Input: part model. Units: mm. Frame: model coordinates. A direction names the side the tool comes from. Give positions to 0.01 mm unless a question says otherwise; leave off trailing zeros. Write each loop counter-clockwise with the first axis right and the second up, starting at its lowest first coordinate (ties: lowest second). Pieces come first, ordered by that corner, then holes. Notation, with made-up numbers: (74, -9) - (111, -9) arc R18 ccw to (111, 9) - close; hole circle Ø11 at (-0.5, 51.5). An arc over 180 degrees is marked (long way). Use a Markdown table: item, result. Add a question column.
1. Section query B-B, the plane z = -95. Return loops of the section in (x, y).
2. Mould query, pull axis X, two halves, no side actions, for faces 5 (the cylindrical face through (-22.2, 12.1, -11.5)), 6 (the cylindrical face through (0.706, 68.675, -112.466)), 7 (the flat face through (-4, 81, -84)). Classes: released by +X, released by -X, zero draft, split by the parting line, or undercut.
3. Section query A-A, the plane x = 0. Return loops of the section in (y, z), plus the area to 3 significant figures.
4. Set-up query: faces 1 (the flat face through (22, 18, 1)), 2 (the flat face through (-22, 18, 1)), 3 (the flat face through (8, 56, -103)), 4 (the flat face through (22, 9, -33.509)). Return all of +Z, -Z, +X, -X, +Y, -Y with unobstructed straight access to the full face (end or side cutting, diameter ignored); none if empty.
5. Section query D-D, the plane y = 73.5. Return loops of the section in (x, z).
6. Material intervals for probe 1 along Z at (x, y) = (14.5, 5); probe 2 along X at (y, z) = (53, -54.5); probe 3 along Y at (x, z) = (-12, -20.5), sorted ascending.
7. Section query C-C, the plane z = -5. Return loops of the section in (x, y), plus the area to 3 significant figures.
8. Pin query (flat end, axial travel): pin 1 (12 mm diameter, centred on x = 19.5, y = 68, fed in from +Z); pin 2 (15.5 mm diameter, centred on x = -22.5, z = -5.51, fed in from -Y); pin 3 (25 mm diameter, centred on x = 19, z = -3, fed in from +Y). Return the tip coordinate at first contact, or that it passes through.
```python
from build123d import *

# Parameters (mm, degrees)
SKETCH1_W           = 56
SKETCH1_H           = 18
BOSS_EXTRUDE1_DEPTH = 75
SKETCH2_R           = 6
CUT_EXTRUDE1_DEPTH  = 75
SKETCH3_W           = 32
SKETCH3_H           = 6
CUT_EXTRUDE2_DEPTH  = 75
BOSS_EXTRUDE5_DEPTH = 6
SKETCH23_R          = 18
SKETCH23_R_2        = 11
BOSS_EXTRUDE7_DEPTH = 25


with BuildPart() as part:
    # Sketch1 → Boss-Extrude1 (new body)
    with BuildSketch(Plane(origin=(0, 0, 0), x_dir=(0, 0, -1), z_dir=(1, 0, 0))):
        with Locations((5.509433962, 9)):
            Rectangle(SKETCH1_W, SKETCH1_H)
    extrude(amount=-BOSS_EXTRUDE1_DEPTH)

    # Sketch2 → Cut-Extrude1 (cut)
    with BuildSketch(Plane(origin=(0, 18, 0), x_dir=(1, 0, 0), z_dir=(0, 1, 0))):
        with Locations(Location((-15, 5.509433962, 0), (0, 0, 270))):
            Circle(SKETCH2_R)
        with Locations(Location((-60, 5.509433962, 0), (0, 0, 270))):
            Circle(SKETCH2_R)
    extrude(amount=-CUT_EXTRUDE1_DEPTH, mode=Mode.SUBTRACT)

    # Sketch3 → Cut-Extrude2 (cut)
    with BuildSketch(Plane(origin=(0, 0, 0), x_dir=(0, 0, -1), z_dir=(1, 0, 0))):
        with Locations((5.509433962, 3)):
            Rectangle(SKETCH3_W, SKETCH3_H)
    extrude(amount=-CUT_EXTRUDE2_DEPTH, mode=Mode.SUBTRACT)


with BuildPart() as part_1:
    # Body-Move/Copy1: moved
    add(part.part.moved(Location((37.5, 0, 0))))

    # Sketch4 → Boss-Extrude5 (add, symmetric)
    with BuildSketch(Plane(origin=(0, 0, 0), x_dir=(0, 0, -1), z_dir=(1, 0, 0))):
        Polygon((65.509433962, 81), (-22.490566038, 18), (33.509433962, 18), (33.509433962, 0), (77.509433962, 56), (77.509433962, 81), align=None)
    extrude(amount=BOSS_EXTRUDE5_DEPTH, both=True)

    # Sketch23 → Boss-Extrude7 (add)
    with BuildSketch(Plane(origin=(0, 81, 0), x_dir=(1, 0, 0), z_dir=(0, 1, 0))):
        with Locations((0, 94.479996711)):
            Circle(SKETCH23_R)
        with Locations(Location((0, 94.479996711, 0), (0, 0, 270))):
            Circle(SKETCH23_R_2, mode=Mode.SUBTRACT)
    extrude(amount=-BOSS_EXTRUDE7_DEPTH)


solid = part_1.part
```
Result sheet:
| question | item | result |
|---|---|---|
| 1 | outline | (-17.99, 56) - (-10.99, 56) - (-10.99, 81) - (-17.99, 81) - close; (10.99, 56) - (17.99, 56) - (17.99, 81) - (10.99, 81) - close |
| 2 | face 5 | undercut |
| 2 | face 6 | split by the parting line |
| 2 | face 7 | zero draft |
| 3 | outline | (0, -33.51) - (56, -77.51) - (56, -83.48) - (81, -83.48) - (81, -65.51) - (18, 22.49) - (0, 22.49) - (0, 10.49) - (6, 10.49) - (6, -21.51) - (0, -21.51) - close; (56, -112.48) - (81, -112.48) - (81, -105.48) - (56, -105.48) - close |
| 3 | area | 4,230 mm² |
| 4 | face 1 | +Z, -Z, +X, +Y |
| 4 | face 2 | +Z, -Z, -X, +Y |
| 4 | face 3 | -Z, +X, -X, -Y |
| 4 | face 4 | -Z, +X, +Y, -Y |
| 5 | outline | (-6, -77.51) arc R18 ccw (long way) to (6, -77.51) - (6, -55.03) - (-6, -55.03) - close; hole circle Ø22 at (0, -94.48) |
| 6 | probe 1 | z = -33.51 to -21.51, 10.49 to 22.49 |
| 6 | probe 2 | x = -6 to 6 |
| 6 | probe 3 | y = 6 to 18 |
| 7 | outline | (-37.5, 6) - (-28.48, 6) - (-28.48, 18) - (-37.5, 18) - close; (-16.52, 6) - (16.52, 6) - (16.52, 18) - (6, 18) - (6, 37.68) - (-6, 37.68) - (-6, 18) - (-16.52, 18) - close; (28.48, 6) - (37.5, 6) - (37.5, 18) - (28.48, 18) - close |
| 7 | area | 849 mm² |
| 8 | pin 1 | stops at z = -82.57 |
| 8 | pin 2 | stops at y = 6 |
| 8 | pin 3 | stops at y = 18 |
